Source: CAD feature listing. Evaluate the final solid. Frame: model axes, mm. A direction names the side the tool comes from. Give positions to 0.01 mm unless a question says otherwise; leave off trailing zeros. Write each loop counter-clockwise with the first axis right and the second up, starting at its lowest first coordinate (ties: lowest second). Pieces come first, ordered by that corner, then holes. Notation, with made-up numbers: (74.5, -36) -> (80.5, -36) arc R23 cw to (80.5, -18) -> close; hole circle Ø9 at (-9.75, -29). An arc over 180 degrees is marked (long way). Write item = value, one per line.
from build123d import *

# Parameters (mm, degrees)
SKETCH_1_W          = 25
SKETCH_1_H          = 30
EXTRUDE_1_DEPTH     = 1
SKETCH_2_W          = 25
SKETCH_2_H          = 25
EXTRUDE_2_DEPTH     = 4
SKETCH_3_R          = 1
CUT_EXTRUDE_1_DEPTH = 1


with BuildPart() as part:
    # 草图1 → 凸台-拉伸1 (new body)
    with BuildSketch(Plane(origin=(0, 0, 0), x_dir=(1, 0, 0), z_dir=(0, 1, 0))):
        Rectangle(SKETCH_1_W, SKETCH_1_H)
    extrude(amount=EXTRUDE_1_DEPTH)

    # 草图2 → 凸台-拉伸2 (add)
    with BuildSketch(Plane(origin=(0, 1, 0), x_dir=(1, 0, 0), z_dir=(0, 1, 0))):
        with Locations((0, 2.5)):
            Rectangle(SKETCH_2_W, SKETCH_2_H)
    extrude(amount=EXTRUDE_2_DEPTH)

    # 草图3 → 切除-拉伸1 (cut)
    with BuildSketch(Plane(origin=(0, 1, 0), x_dir=(1, 0, 0), z_dir=(0, 1, 0))):
        with Locations(Location((-11.1, -13.6, 0), (0, 0, 270))):
            Circle(SKETCH_3_R)
        with Locations(Location((11.1, -13.6, 0), (0, 0, 270))):
            Circle(SKETCH_3_R)
    extrude(amount=-CUT_EXTRUDE_1_DEPTH, mode=Mode.SUBTRACT)


solid = part.part
(1) Section query C-C (x = -5.5). Return loops of the section in (y, z).
Values follow:
outline = (0, -15) -> (5, -15) -> (5, 10) -> (1, 10) -> (1, 15) -> (0, 15) -> close
(2) First-contact query: pin 1 (5.5 mm diameter, centred on x = 2, z = 13, fed in from +Y). Flat tip, straight axial feed; report the tip coordinate or a pass-through.
Values follow:
pin_1 = 1
(3) Pull-direction query (Z, two-part tool) for faces 1 (the face through (0, 3, 10)), 2 (the face through (0, 5, -3)), 3 (the face through (-10.8, 0.507, 14.554)); classes: pulls with the +Z half, pulls with the -Z half, needs draft (parallel to the pull), parting line crosses it, or undercut.
Values follow:
face_1 = pulls with the +Z half
face_2 = needs draft
face_3 = undercut
(4) Material intervals for line 1 (X direction, y = 0.75, z = 13.6); line 2 (Z direction, x = 6.5, y = 1.45); line 3 (Y direction, x = 9.5, z = 11.25), sorted ascending.
Values follow:
line_1 = -12.5 to -12.1, -10.1 to 10.1, 12.1 to 12.5
line_2 = -15 to 10
line_3 = 0 to 1
(5) Access query for faces 4 (the face through (0, 0, 0)), 5 (the face through (0, 1, 12)). Directions: +Z, -Z, +X, -X, +Y, -Y. A direction counts if a zero-diameter tool reaches every point of the face in a straight line with its end or side. Return the directions, or none.
Values follow:
face_4 = +Z, -Z, +X, -X, -Y
face_5 = +Z, +X, -X, +Y
(6) Section query D-D (y = 3.95). Return loops of the section in (x, z), plus the area to 3 significant figures.
Values follow:
outline = (-12.5, -15) -> (12.5, -15) -> (12.5, 10) -> (-12.5, 10) -> close
area = 625 mm2
(7) Section query A-A (x = -11.1). Return loops of the section in (y, z), plus the area to 3 significant figures.
Values follow:
outline = (0, -15) -> (5, -15) -> (5, 10) -> (1, 10) -> (1, 12.6) -> (0, 12.6) -> close; (0, 14.6) -> (1, 14.6) -> (1, 15) -> (0, 15) -> close
area = 128 mm2
(8) Section query B-B (z = 13.6). Return loops of the section in (x, y), plus the area to 3 significant figures.
Values follow:
outline = (-12.5, 0) -> (-12.1, 0) -> (-12.1, 1) -> (-12.5, 1) -> close; (-10.1, 0) -> (10.1, 0) -> (10.1, 1) -> (-10.1, 1) -> close; (12.1, 0) -> (12.5, 0) -> (12.5, 1) -> (12.1, 1) -> close
area = 21.0 mm2
